Geometry check sheet. Reference: the model listing, model coordinates, mm. Round coordinates to 2 decimals unless told otherwise and drop trailing zeros. Loops run counter-clockwise (first coordinate to the right, second up) from the corner with the lowest first, then second, coordinate; pieces in that order, holes last. Notation, with made-up numbers: M -30.75,2 L 10.25,2 A12 ccw 10.25,7 Z; hole C -21.75,87 d1. An arc over 180 degrees is marked long. Write item = value, one per line.
from build123d import *

# Parameters (mm, degrees)
SKETCH1_R           = 50
SKETCH1_R_2         = 5
BOSS_EXTRUDE1_DEPTH = 1.59
SKETCH2_R           = 1.75
CUT_EXTRUDE1_DEPTH  = 1.59
SKETCH3_R           = 1.5
CUT_EXTRUDE2_DEPTH  = 10


with BuildPart() as part:
    # Sketch1 → Boss-Extrude1 (new body)
    with BuildSketch(Plane.XY):
        with Locations(Location((0, 0, 0), (0, 0, 180))):
            Circle(SKETCH1_R)
        with Locations(Location((0, 0, 0), (0, 0, 180))):
            Circle(SKETCH1_R_2, mode=Mode.SUBTRACT)
    extrude(amount=BOSS_EXTRUDE1_DEPTH)

    # Sketch2 → Cut-Extrude1 (cut)
    with BuildSketch(Plane.XY.offset(1.59)):
        with Locations((0, 45)):
            Circle(SKETCH2_R)
        with Locations((45, 0)):
            Circle(SKETCH2_R)
        with Locations((0, -45)):
            Circle(SKETCH2_R)
        with Locations((-45, 0)):
            Circle(SKETCH2_R)
    extrude(amount=-CUT_EXTRUDE1_DEPTH, mode=Mode.SUBTRACT)

    # Sketch3 → Cut-Extrude2 (cut)
    with BuildSketch(Plane.XY.offset(1.59)):
        with Locations((-27.86, 27.860014357)):
            Circle(SKETCH3_R)
        with Locations((27.860014357, 27.86)):
            Circle(SKETCH3_R)
        with Locations((27.86, -27.860014357)):
            Circle(SKETCH3_R)
        with Locations((-27.860014357, -27.86)):
            Circle(SKETCH3_R)
    extrude(amount=-CUT_EXTRUDE2_DEPTH, mode=Mode.SUBTRACT)


solid = part.part
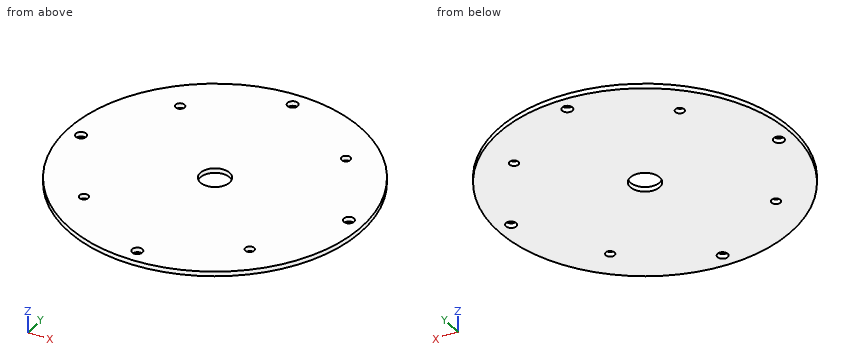
(1) Sectioned sample at C-C on x = -45. Record the cut outline in (y, z).
Result set:
outline = M -21.79,0 L -1.75,0 L -1.75,1.59 L -21.79,1.59 Z; M 1.75,0 L 21.79,0 L 21.79,1.59 L 1.75,1.59 Z
(2) Depth check by flat-ended pin: pin 1 Ø3 at (x, y) = (31, 5) entering from -Z; pin 2 Ø2.5 at (x, y) = (27.86, 27.86) entering from -Z. Enter the tip coordinate at first touch or a pass-through.
Result set:
pin_1 = 0
pin_2 = through
(3) Sectioned sample at D-D on z = 0.55. State how many separate pieces and enclosed holes the cut face has, then the cut area to 3 significant figures.
Result set:
separate_pieces = 1
enclosed_holes = 9
area = 7,710 mm2
(4) Sectioned sample at A-A on x = 0. Record the cut outline in (y, z).
Result set:
outline = M -50,0 L -46.75,0 L -46.75,1.59 L -50,1.59 Z; M -43.25,0 L -5,0 L -5,1.59 L -43.25,1.59 Z; M 5,0 L 43.25,0 L 43.25,1.59 L 5,1.59 Z; M 46.75,0 L 50,0 L 50,1.59 L 46.75,1.59 Z
(5) Material ranges on line 1 along Y through (x, z) = (0, 1.3); line 2 along X through (y, z) = (-29, 0.5); line 3 along Y through (x, z) = (-27.86, 0.85), recorded low to high. Write a range as from..to.
Result set:
line_1 = -50..-46.75, -43.25..-5, 5..43.25, 46.75..50
line_2 = -40.73..-28.83, -26.89..26.89, 28.83..40.73
line_3 = -41.52..-29.36, -26.36..26.36, 29.36..41.52
